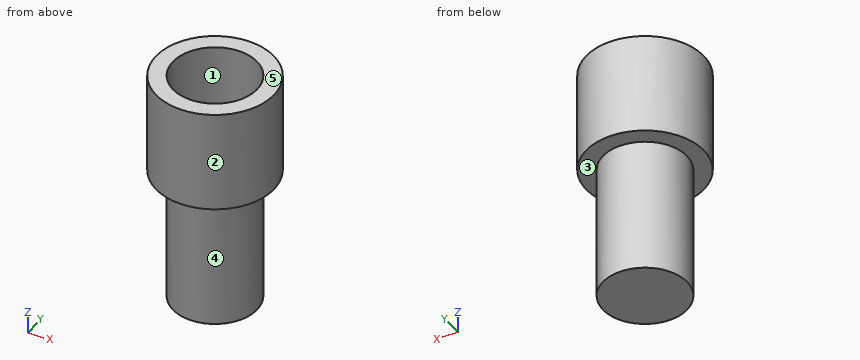
```python
from build123d import *

# Parameters (mm, degrees)
ESQUISSE1_R             = 3.5
BOSS_EXTRU_2_DEPTH      = 6
ESQUISSE3_R             = 2.5
ENL_V_MAT_EXTRU_1_DEPTH = 5
ESQUISSE4_R             = 2.5
BOSS_EXTRU_3_DEPTH      = 8


with BuildPart() as part:
    # Esquisse1 → Boss.-Extru.2 (new body)
    with BuildSketch(Plane.XY):
        Circle(ESQUISSE1_R)
    extrude(amount=BOSS_EXTRU_2_DEPTH)

    # Esquisse3 → Enlèv. mat.-Extru.1 (cut)
    with BuildSketch(Plane.XY.offset(6)):
        Circle(ESQUISSE3_R)
    extrude(amount=-ENL_V_MAT_EXTRU_1_DEPTH, mode=Mode.SUBTRACT)

    # Esquisse4 → Boss.-Extru.3 (add)
    with BuildSketch(Plane(origin=(0, 0, 0), x_dir=(-1, 0, 0), z_dir=(0, 0, -1))):
        with Locations(Location((0, 0, 0), (0, 0, 180))):
            Circle(ESQUISSE4_R)
    extrude(amount=BOSS_EXTRU_3_DEPTH)


solid = part.part
```
Check sheet for the modelled part. Datum: model origin and axes. Units: mm. Face numbers are marked on the shaded views. A direction names the side the tool comes from. Round coordinates to 2 decimals unless told otherwise and drop trailing zeros. Loops run counter-clockwise (first coordinate to the right, second up) from the corner with the lowest first, then second, coordinate; pieces in that order, holes last. Notation, with made-up numbers: (22, 57) -> (38, 57) arc R17 cw to (38, 81) -> close; hole circle Ø1 at (8.25, 66.25). An arc over 180 degrees is marked (long way). Write item = value, one per line. Start each with the question number.
1) Sectioned sample at C-C, the plane z = 1.5. Record the cut outline in (x, y).
2) Set-up check for the marked faces 4 and 5: record each of +Z, -Z, +X, -X, +Y, -Y from which the full face is reachable in a straight line by a thin tool's end or side.
3) Sectioned sample at A-A, the plane y = 0. Record the cut outline in (x, z).
4) Gauge pin test, flat ends, axial feed: pin 1 Ø1 at (y, z) = (2, 1.5) entering from -X; pin 2 Ø2 at (x, z) = (-1, -2.5) entering from -Y; pin 3 Ø2.5 at (x, y) = (0.5, -0.5) entering from +Z. Record the tip position at first contact, or that the pin passes through.
5) Thickness scan on probe 1 along Y at (x, z) = (0, 2.7); probe 2 along Z at (x, y) = (-0.5, 0.5); probe 3 along Z at (x, y) = (-0.75, -2.5). Record the ranges inside material, lowest first.
6) Sectioned sample at D-D, the plane z = -3.5. Record the cut outline in (x, y), plus the area to 3 significant figures.
7) Release check for a two-part mould opening along Y. For the marked faces 1, 2 and 3 record: released by +Y, released by -Y, zero draft, split by the parting line, or undercut.
Results are:
q1.outline = circle Ø7 at (0, 0); hole circle Ø5 at (0, 0)
q2.face_4 = -Z
q2.face_5 = +Z, +X, -X, +Y, -Y
q3.outline = (-3.5, 0) -> (-2.5, 0) -> (-2.5, -8) -> (2.5, -8) -> (2.5, 0) -> (3.5, 0) -> (3.5, 6) -> (2.5, 6) -> (2.5, 1) -> (-2.5, 1) -> (-2.5, 6) -> (-3.5, 6) -> close
q4.pin_1 = -3.16
q4.pin_2 = -2.5
q4.pin_3 = 1
q5.probe_1 = -3.5 to -2.5, 2.5 to 3.5
q5.probe_2 = -8 to 1
q5.probe_3 = 0 to 6
q6.outline = circle Ø5 at (0, 0)
q6.area = 19.6 mm^2
q7.face_1 = undercut
q7.face_2 = split by the parting line
q7.face_3 = zero draft
